Design review of the part built by this model. Coordinates are the model's own, in mm. A direction names the side the tool comes from. Give positions to 0.01 mm unless a question says otherwise; leave off trailing zeros. Order: outer loops, then holes, each group sorted by start corner. A loop starts at its lowest first (then second) coordinate and runs counter-clockwise, first axis right, second up.
```python
from build123d import *

# Parameters (mm, degrees)
F1_DEPTH = 25.4
F3_D     = 15.24
F4_SIZE  = 5.08


with BuildPart() as f1:
    # F0 (on Right) → F1 (new body)
    with BuildSketch(Plane.YZ):
        Polygon((0, 46.745047), (0, 0), (22.818567, 0), (22.818567, 17.724711), (45.616407, 17.724711), (45.616407, 46.745047), align=None)
    extrude(amount=F1_DEPTH)

    # F3 (through all)
    with Locations(Plane.YZ.offset(25.4)):
        with Locations((15.24, 31.505047)):
            Hole(F3_D / 2)

    # F4
    f4_edges = [f1.edges().sort_by_distance(p)[0] for p in [
        (12.7, 45.616407, 17.724711),
        (0, 45.616407, 32.234879),
        (12.7, 45.616407, 46.745047),
        (25.4, 45.616407, 32.234879),
    ]]
    chamfer(f4_edges, length=F4_SIZE)


solid = f1.part
```
1. For pin 1 (9 mm diameter, centred on x = 14, y = 28.5, fed in from -Z); pin 2 (5.5 mm diameter, centred on x = 10, z = 5.5, fed in from +Y), all flat-tipped, find the tip position at first contact; note any pin that passes through.
Recorded:
pin 1: stops at z = 17.72
pin 2: stops at y = 22.82
2. Take a section at C-C (x = 2.75). State the section outline as (y, z) points, then the cut area to 3 significant figures.
Recorded:
outline: (0, 0) - (22.82, 0) - (22.82, 17.72) - (40.54, 17.72) - (43.29, 20.47) - (43.29, 44) - (40.54, 46.75) - (0, 46.75) - close; hole circle Ø15.24 at (15.24, 31.51)
area: 1,470 mm2
3. For line 1 along Z through (x, y) = (5.5, 15.24); line 2 along Y through (x, z) = (18.25, 16.5); line 3 along Z through (x, y) = (2.25, 21), list the stretches that pass through material, from the lowest coordinate up.
Recorded:
line 1: z = 0 to 23.89, 39.13 to 46.75
line 2: y = 0 to 22.82
line 3: z = 0 to 26.52, 36.49 to 46.75
4. Take a section at A-A (y = 15.24). State the section outline as (x, z) points, then the cut area to 3 significant figures.
Recorded:
outline: (0, 0) - (25.4, 0) - (25.4, 23.89) - (0, 23.89) - close; (0, 39.13) - (25.4, 39.13) - (25.4, 46.75) - (0, 46.75) - close
area: 800 mm2
5. Take a section at D-D (y = 26). State the section outline as (x, z) points, then the cut area to 3 significant figures.
Recorded:
outline: (0, 17.72) - (25.4, 17.72) - (25.4, 46.75) - (0, 46.75) - close
area: 737 mm2
6. Machinability: for faces 4 (the face through (12.52, 43.11, 44.17)), 5 (the face through (13, 22.819, 9)), which of the approach directions +Z, -Z, +X, -X, +Y, -Y give a long, thin tool a straight path to every point of the face, cutting with its end or side? Answer none if there is none.
Recorded:
face 4: +Z, +X, -X, +Y
face 5: -Z, +X, -X, +Y
7. Take a section at B-B (z = 25.5). State the section outline as (x, y) points, then the cut area to 3 significant figures.
Recorded:
outline: (0, 0) - (25.4, 0) - (25.4, 10.55) - (0, 10.55) - close; (0, 19.93) - (25.4, 19.93) - (25.4, 40.54) - (20.32, 45.62) - (5.08, 45.62) - (0, 40.54) - close
area: 895 mm2
8. Draft analysis for pull direction Z (two halves, no side actions). For faces 1 (the face through (13, 11, 0)), 2 (the face through (12.52, 7.97, 33.79)), 3 (the face through (13, 0, 24)), state which applies: pulls with the +Z half, pulls with the -Z half, needs draft (parallel to the pull), parting line crosses it, or undercut.
Recorded:
face 1: pulls with the -Z half
face 2: undercut
face 3: needs draft
